Design review of the part shown in the three views and the two pictorial views. Dimensions are in mm from the part's minimum x, y and z. Give positions to 0.01 mm unless a question says otherwise; leave off trailing zeros. Order: outer loops, then holes, each group sorted by start corner. A loop starts at its lowest first (then second) coordinate and runs counter-clockwise, first axis right, second up. Notation, with made-up numbers: (8, 39) -> (66, 39) arc R9 ccw to (66, 51) -> close; hole circle Ø8 at (32, -5). An arc over 180 degrees is marked (long way). Answer in a Markdown table with one row per item. Add a question column.
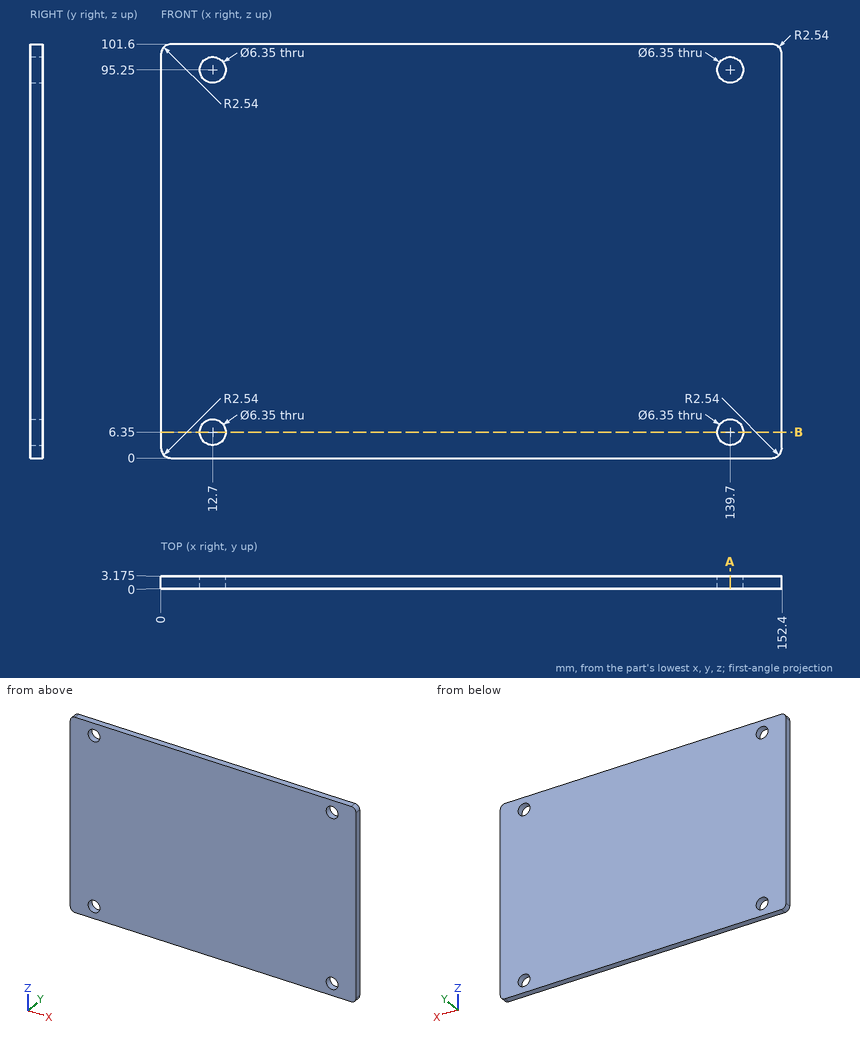
1) Add section B-B, the plane z = 6.35. Write out the cut boundary in (x, y) (3 decimals).
2) For L1, parallel to X at y = 2.1, z = 95.25 (3 decimals); L2, parallel to Z at x = 139.7, y = 1.35 (3 decimals); L3, parallel to Z at x = 137.5, y = 1.1, list the stretches that pass through material, from the lowest coordinate up.
3) Add section A-A, the plane x = 139.7. Write out the cut boundary in (y, z) (3 decimals), and give its area (3 significant figures).
4) Clearance check with a flat-ended pin moving along its axis: P1, Ø5, axis at x = 139.7, z = 95.25, coming from the -Y side. State where the tip first meets the part, or that it passes through.
Verdict:
| question | item | result |
|---|---|---|
| 1 | outline | (0, 0) -> (9.525, 0) -> (9.525, 3.175) -> (0, 3.175) -> close; (15.875, 0) -> (136.525, 0) -> (136.525, 3.175) -> (15.875, 3.175) -> close; (142.875, 0) -> (152.4, 0) -> (152.4, 3.175) -> (142.875, 3.175) -> close |
| 2 | L1 | x = 0 to 9.525, 15.875 to 136.525, 142.875 to 152.4 |
| 2 | L2 | z = 0 to 3.175, 9.525 to 92.075, 98.425 to 101.6 |
| 2 | L3 | z = 0 to 4.06, 8.64 to 92.96, 97.54 to 101.6 |
| 3 | outline | (0, 0) -> (3.175, 0) -> (3.175, 3.175) -> (0, 3.175) -> close; (0, 9.525) -> (3.175, 9.525) -> (3.175, 92.075) -> (0, 92.075) -> close; (0, 98.425) -> (3.175, 98.425) -> (3.175, 101.6) -> (0, 101.6) -> close |
| 3 | area | 282 mm2 |
| 4 | P1 | passes through |
